```python
from build123d import *

# Parameters (mm, degrees)
F0_W     = 104.775
F0_H     = 104.775
F1_DEPTH = 50.8
F2_W     = 34.036
F2_H     = 19.685
F3_DEPTH = 104.775
F4_W     = 34.036
F4_H     = 19.6899231523
F4_H_2   = 19.685
F5_DEPTH = 158.242


with BuildPart() as f1:
    # F0 (on Top) → F1 (new body)
    with BuildSketch(Plane.XY):
        with Locations((52.3875, 52.3875)):
            Rectangle(F0_W, F0_H)
    extrude(amount=F1_DEPTH)

    # F2 (on face) → F3 (cut)
    with BuildSketch(Plane.XZ):
        with Locations((87.757, 40.9575)):
            Rectangle(F2_W, F2_H)
        with Locations((17.018, 40.9575)):
            Rectangle(F2_W, F2_H)
    extrude(amount=-F3_DEPTH, mode=Mode.SUBTRACT)

    # F4 (on Right) → F5 (cut)
    with BuildSketch(Plane.YZ):
        with Locations((89.075582438, 9.8449615762)):
            Rectangle(F4_W, F4_H)
        with Locations((17.018, 9.8425)):
            Rectangle(F4_W, F4_H_2)
    extrude(amount=F5_DEPTH, mode=Mode.SUBTRACT)


solid = f1.part
```
Model file for the job. Use its own axes, mm. A direction names the side the tool comes from. Give positions to 0.01 mm unless a question says otherwise; leave off trailing zeros. Write each loop counter-clockwise with the first axis right and the second up, starting at its lowest first coordinate (ties: lowest second). Pieces come first, ordered by that corner, then holes. Notation, with made-up numbers: (-39.5, 69) - (-26.5, 69) arc R17 ccw to (-26.5, 78) - close; hole circle Ø4 at (-2.5, 23.25). An arc over 180 degrees is marked (long way). One line per question, with ' | ' between items. Start each with the question number.
(1) Slice it at C-C on z = 4.5. Write the cut outline in (x, y) (3 decimals).
(2) Wall check: line 1 along Y through (x, z) = (62.5, 6); line 2 along Z through (x, y) = (78, 48.5) (3 decimals); line 3 along X through (y, z) = (75, 39). Give the ranges that are in metal, low to high. Write a range as from..to.
(3) Slice it at B-B on x = 25. Write the cut outline in (y, z) (3 decimals).
(4) 3-axis set-ups, long thin cutter, end or side, ignore diameter. For faces 1 (the face through (34.036, 52, 41)), 2 (the face through (52, 53, 0)), 3 (the face through (70.739, 52, 41)), 4 (the face through (52, 17, 19.685)), 5 (the face through (52, 72.058, 10)): which of +Z, -Z, +X, -X, +Y, -Y reach the whole face in a straight line?
(5) Slice it at A-A on y = 61. Write the cut outline in (x, z) (3 decimals).
(6) Pin check, flat tips, straight feed: P1, Ø10, axis at y = 33.5, z = 45.5, coming from the -X side; P2, Ø17, axis at x = 19.5, y = 69.5, coming from the +Z side (3 decimals); P3, Ø6, axis at y = 75.5, z = 9.5, coming from the -X side; P4, Ø15.5, axis at y = 67, z = 40, coming from the +X side. Stop position of each tip, or through.
(7) Slice it at D-D on z = 33. Write the cut outline in (x, y) (3 decimals).
Results below:
1) outline: (0, 34.036) - (104.775, 34.036) - (104.775, 72.058) - (0, 72.058) - close
2) line 1: 34.04..72.06 | line 2: 0..31.115 | line 3: 34.04..70.74
3) outline: (0, 19.685) - (34.036, 19.685) - (34.036, 0) - (72.058, 0) - (72.058, 19.69) - (104.775, 19.69) - (104.775, 31.115) - (0, 31.115) - close
4) face 1: +Z, -X, +Y, -Y | face 2: -Z, +X, -X, +Y, -Y | face 3: +Z, +X, +Y, -Y | face 4: -Z, +X, -X, -Y | face 5: -Z, +X, -X, +Y
5) outline: (0, 0) - (104.775, 0) - (104.775, 31.115) - (70.739, 31.115) - (70.739, 50.8) - (34.036, 50.8) - (34.036, 31.115) - (0, 31.115) - close
6) P1: x = 34.04 | P2: z = 31.115 | P3: through | P4: x = 70.74
7) outline: (34.036, 0) - (70.739, 0) - (70.739, 104.775) - (34.036, 104.775) - close
